Here's the drawing with two shaded views (mm, measured from the low corner). I have some questions. A direction names the side the tool comes from. Give positions to 0.01 mm unless a question says otherwise; leave off trailing zeros. Loops run counter-clockwise (first coordinate to the right, second up) from the corner with the lowest first, then second, coordinate; pieces in that order, holes last. Notation, with made-up numbers: (48.25, 84) -> (60.25, 84) arc R15 ccw to (60.25, 112) -> close; hole circle Ø6 at (9, -9.75). An arc over 180 degrees is marked (long way). Write each question's results on one line, items separated by ' | '. Start each with the question number.
Q1. If we section it at A-A, the plane z = 16.51: List the corners of the cut face in (x, y) for me.
Q2. Will these pins go through, and if not, where does the flat tip stop? P1, Ø4, axis at x = 49, z = 23.5, coming from the -Y side; P2, Ø1.5, axis at x = 40, y = 1, coming from the -Z side.
Q3. If we section it at C-C, the plane y = 4.8: List the corners of the cut face in (x, z) for me.
Q4. If we section it at B-B, the plane x = 35: List the corners of the cut face in (y, z) for me.
Q5. If I drill on line 1 along X through (y, z) = (5.2, 16.51); line 2 along Y through (x, z) = (13, 16); line 3 along Z through (x, y) = (40, 3.25), over which ranges is the centre line in solid material (lowest first)?
Q6. If we section it at D-D, the plane x = 62.5: List the corners of the cut face in (y, z) for me.
Q7. Which directions (+Z, -Z, +X, -X, +Y, -Y) give clear straight access to the entire face, cutting with the end or side of a thin tool? Please do the marked faces 1 and 2.
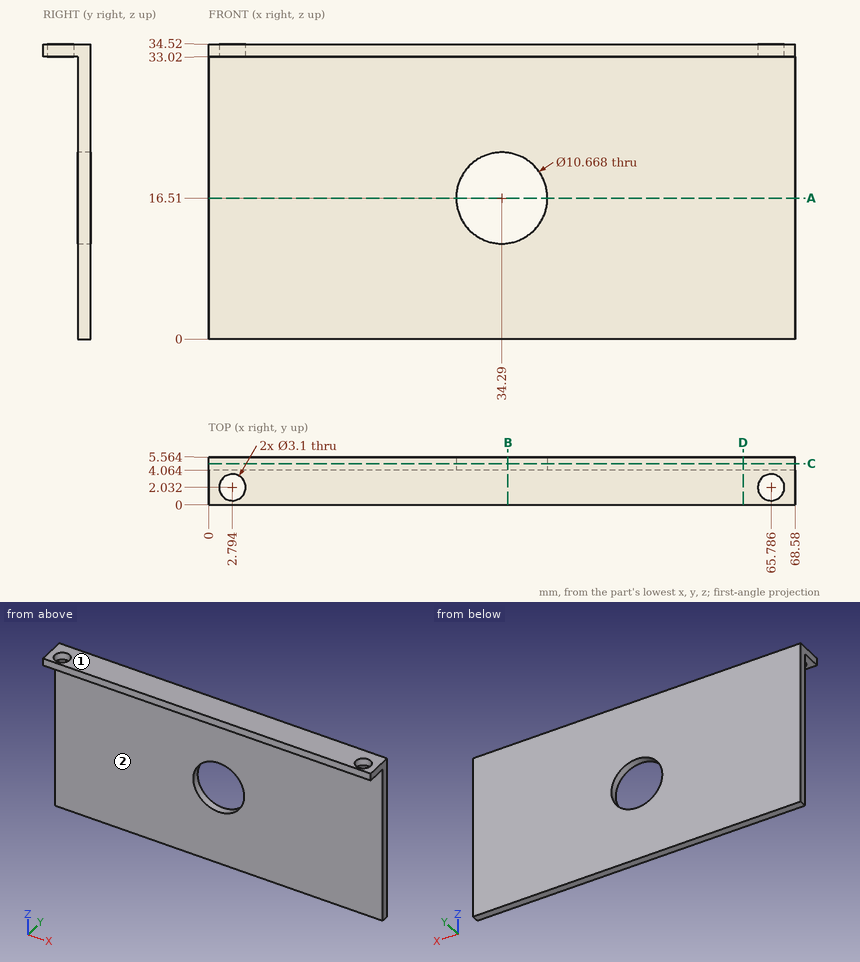
Final values:
1) outline: (0, 4.06) -> (28.96, 4.06) -> (28.96, 5.56) -> (0, 5.56) -> close; (39.62, 4.06) -> (68.58, 4.06) -> (68.58, 5.56) -> (39.62, 5.56) -> close
2) P1: stops at y = 4.06 | P2: stops at z = 33.02
3) outline: (0, 0) -> (68.58, 0) -> (68.58, 34.52) -> (0, 34.52) -> close; hole circle Ø10.67 at (34.29, 16.51)
4) outline: (0, 33.02) -> (4.06, 33.02) -> (4.06, 21.8) -> (5.56, 21.8) -> (5.56, 34.52) -> (0, 34.52) -> close; (4.06, 0) -> (5.56, 0) -> (5.56, 11.22) -> (4.06, 11.22) -> close
5) line 1: x = 0 to 28.96, 39.62 to 68.58 | line 2: y = 4.06 to 5.56 | line 3: z = 33.02 to 34.52
6) outline: (0, 33.02) -> (4.06, 33.02) -> (4.06, 0) -> (5.56, 0) -> (5.56, 34.52) -> (0, 34.52) -> close
7) face 1: +Z, +X, -X, +Y, -Y | face 2: -Z, +X, -X, -Y
